```python
from build123d import *

# Parameters (mm, degrees)
SKETCH1_W            = 64
SKETCH1_H            = 16
BOSS_EXTRUDE1_DEPTH  = 9.6
SKETCH2_R            = 2.4
BOSS_EXTRUDE2_DEPTH  = 1.6
LPATTERN1_COUNT      = 8
LPATTERN1_PITCH      = 8
LPATTERN1_COUNT_DIR2 = 2
LPATTERN1_PITCH_DIR2 = 8
SHELL1_T             = -1.6
SKETCH3_R            = 3.256
SKETCH3_R_2          = 2.4
BOSS_EXTRUDE3_DEPTH  = 8
LPATTERN2_COUNT      = 7
LPATTERN2_PITCH      = 8


with BuildPart() as part:
    # Sketch1 → Boss-Extrude1 (new body)
    with BuildSketch(Plane.XY):
        with Locations((32, 8)):
            Rectangle(SKETCH1_W, SKETCH1_H)
    extrude(amount=BOSS_EXTRUDE1_DEPTH)

    # Sketch2 → Boss-Extrude2 (add)
    with BuildSketch(Plane.XY.offset(9.6)):
        with Locations((4, 12)):
            Circle(SKETCH2_R)
    boss_extrude2 = extrude(amount=BOSS_EXTRUDE2_DEPTH)

    # LPattern1: Boss-Extrude2 8 × 2
    with Locations(*[(i * LPATTERN1_PITCH, -j * LPATTERN1_PITCH_DIR2, 0) for i in range(LPATTERN1_COUNT) for j in range(LPATTERN1_COUNT_DIR2) if (i, j) != (0, 0)]):
        add(boss_extrude2)

    # Shell1
    shell1_openings = [part.faces().sort_by_distance(p)[0] for p in [
        (32, 8, 0),
    ]]
    offset(amount=SHELL1_T, openings=shell1_openings, kind=Kind.INTERSECTION)

    # Sketch3 → Boss-Extrude3 (add)
    with BuildSketch(Plane(origin=(0, 0, 8), x_dir=(-1, 0, 0), z_dir=(0, 0, -1))):
        with Locations((-8, 8)):
            Circle(SKETCH3_R)
        with Locations((-8, 8)):
            Circle(SKETCH3_R_2, mode=Mode.SUBTRACT)
    boss_extrude3 = extrude(amount=BOSS_EXTRUDE3_DEPTH)

    # LPattern2: Boss-Extrude3 ×7
    with Locations(*[(i * LPATTERN2_PITCH, 0, 0) for i in range(1, LPATTERN2_COUNT)]):
        add(boss_extrude3)


solid = part.part
```
Input: part model. Units: mm. Frame: model coordinates. A direction names the side the tool comes from. Coordinates: 2 decimals unless noted, no trailing zeros. Write each loop counter-clockwise with the first axis right and the second up, starting at its lowest first coordinate (ties: lowest second). Pieces come first, ordered by that corner, then holes. Notation, with made-up numbers: (24.5, 37) -> (69.5, 37) arc R10 cw to (69.5, 48) -> close; hole circle Ø1 at (-15.75, 0.5). An arc over 180 degrees is marked (long way). Write each question's results on one line, items separated by ' | '.
Item 1: Set-up query: faces 4 (the flat face through (32, 1.6, 4)), 5 (the cylindrical face through (35.69, 14.38, 10.39)), 6 (the flat face through (4, 4, 11.2)). Return all of +Z, -Z, +X, -X, +Y, -Y with unobstructed straight access to the full face (end or side cutting, diameter ignored); none if empty.
Conclusion:
face 4: -Z | face 5: +Z | face 6: +Z, +X, -X, +Y, -Y
Item 2: Mould query, pull axis X, two halves, no side actions, for faces 1 (the flat face through (0, 8, 5)), 2 (the flat face through (20, 12, 9.6)), 3 (the flat face through (20, 12, 11.2)). Classes: +X half, -X half, draft (parallel to the pull), parting line (faces both ways), or undercut.
Conclusion:
face 1: -X half | face 2: undercut | face 3: draft
Item 3: Section query C-C on y = 15. Return loops of the section in (x, z), plus the area to 3 significant figures.
Conclusion:
outline: (0, 0) -> (64, 0) -> (64, 9.6) -> (0, 9.6) -> close | area: 614 mm^2
Item 4: Section query A-A on z = 2.25. Count the separate pieces of the cut face and the enclosed holes in it, plus the area to 3 significant figures.
Conclusion:
separate pieces: 8 | enclosed holes: 8 | area: 352 mm^2
Item 5: Material intervals for probe 1 along Y at (x, z) = (32, 2.5); probe 2 along Y at (x, z) = (52, 8.85); probe 3 along X at (y, z) = (3.5, 5), sorted ascending.
Conclusion:
probe 1: y = 0 to 1.6, 4.74 to 5.6, 10.4 to 11.26, 14.4 to 16 | probe 2: y = 0 to 3.2, 4.8 to 11.2, 12.8 to 16 | probe 3: x = 0 to 1.6, 62.4 to 64
Item 6: Section query D-D on x = 56. Return loops of the section in (y, z), plus the area to 3 significant figures.
Conclusion:
outline: (0, 0) -> (1.6, 0) -> (1.6, 8) -> (4.74, 8) -> (4.74, 0) -> (5.6, 0) -> (5.6, 8) -> (10.4, 8) -> (10.4, 0) -> (11.26, 0) -> (11.26, 8) -> (14.4, 8) -> (14.4, 0) -> (16, 0) -> (16, 9.6) -> (0, 9.6) -> close | area: 64.9 mm^2
Item 7: Section query B-B on x = 12. Return loops of the section in (y, z), plus the area to 3 significant figures.
Conclusion:
outline: (0, 0) -> (1.6, 0) -> (1.6, 8) -> (3.2, 8) -> (3.2, 9.6) -> (4.8, 9.6) -> (4.8, 8) -> (11.2, 8) -> (11.2, 9.6) -> (12.8, 9.6) -> (12.8, 8) -> (14.4, 8) -> (14.4, 0) -> (16, 0) -> (16, 9.6) -> (14.4, 9.6) -> (14.4, 11.2) -> (9.6, 11.2) -> (9.6, 9.6) -> (6.4, 9.6) -> (6.4, 11.2) -> (1.6, 11.2) -> (1.6, 9.6) -> (0, 9.6) -> close | area: 61.4 mm^2
Item 8: Pin query (flat end, axial travel): pin 1 Ø1.8 at (x, y) = (60.5, 4) entering from -Z; pin 2 Ø3 at (x, y) = (16, 8) entering from +Z; pin 3 Ø1.3 at (x, y) = (60, 4) entering from -Z. Return the tip coordinate at first contact, or that it passes through.
Conclusion:
pin 1: stops at z = 8 | pin 2: stops at z = 9.6 | pin 3: stops at z = 9.6
